```python
from build123d import *

# Parameters (mm, degrees)
SKETCH1_R               = 67
SKETCH1_R_2             = 2.5
BOSS_EXTRUDE1_DEPTH     = 6
CUT_EXTRUDE3_DEPTH      = 47
CUT_EXTRUDE3_DEPTH_BACK = 25
CUT_EXTRUDE6_DEPTH      = 10
CUT_EXTRUDE7_DEPTH      = 10


with BuildPart() as part:
    # Sketch1 → Boss-Extrude1 (new body)
    with BuildSketch(Plane.XY):
        Circle(SKETCH1_R)
        with Locations((0, 58)):
            Circle(SKETCH1_R_2, mode=Mode.SUBTRACT)
        with Locations((58, 0)):
            Circle(SKETCH1_R_2, mode=Mode.SUBTRACT)
        with Locations((0, -58)):
            Circle(SKETCH1_R_2, mode=Mode.SUBTRACT)
        with Locations((-58, 0)):
            Circle(SKETCH1_R_2, mode=Mode.SUBTRACT)
    extrude(amount=BOSS_EXTRUDE1_DEPTH)

    # Sketch3 → Cut-Extrude3 (cut, two sides: drawn at the far end of the back side and taken through both)
    with BuildSketch(Plane.XY.offset(6).offset(-CUT_EXTRUDE3_DEPTH_BACK)):
        Polygon((-34.424621456, -26.646446356), (-27.353553137, -19.575379051), (-19.575378544, -27.353553644), (-26.646446863, -34.424620949), align=None)
        Polygon((19.575379051, 27.353553137), (27.353553644, 19.575378544), (34.424620949, 26.646446863), (26.646446356, 34.424621456), align=None)
    extrude(amount=CUT_EXTRUDE3_DEPTH + CUT_EXTRUDE3_DEPTH_BACK, mode=Mode.SUBTRACT)

    # Sketch4 → Cut-Extrude6 (cut)
    with BuildSketch(Plane.XY.offset(6)):
        Polygon((-19.445436483, 33.587572106), (33.587572106, -19.445436483), (19.445436483, -33.587572106), (-33.587572106, 19.445436483), align=None)
    extrude(amount=-CUT_EXTRUDE6_DEPTH, mode=Mode.SUBTRACT)

    # Sketch5 → Cut-Extrude7 (cut)
    with BuildSketch(Plane.XY.offset(6)):
        Polygon((-34.424621456, -26.646446356), (-34.778174339, -26.292893473), (-27.707106527, -19.221825661), (-27.353553137, -19.575379051), align=None)
        Polygon((-26.646446863, -34.424620949), (-26.292893473, -34.778174339), (-19.221825661, -27.707106527), (-19.575378544, -27.353553644), align=None)
        Polygon((27.707106527, 19.221825661), (27.353553644, 19.575378544), (34.424620949, 26.646446863), (34.778174339, 26.292893473), align=None)
        Polygon((26.646446356, 34.424621456), (19.575379051, 27.353553137), (19.221825661, 27.707106527), (26.292893473, 34.778174339), align=None)
    extrude(amount=-CUT_EXTRUDE7_DEPTH, mode=Mode.SUBTRACT)


solid = part.part
```
The listing builds one solid part. Answer for the finished solid, in the listing's coordinates (mm). A direction names the side the tool comes from. Coordinates: 2 decimals unless noted, no trailing zeros. Loops run counter-clockwise (first coordinate to the right, second up) from the corner with the lowest first, then second, coordinate; pieces in that order, holes last. Notation, with made-up numbers: M 7,-20 L 20,-20 A26 cw 20,5 Z; hole C -23,-40 d8. An arc over 180 degrees is marked long. Answer as CSV lines item,"result". Start each with the question number.
(1) Given pin 1 (2 mm diameter, centred on y = 44, z = 3.5, fed in from +X); pin 2 (1.5 mm diameter, centred on y = -51, z = 5, fed in from +X); pin 3 (1 mm diameter, centred on y = -29, z = 5, fed in from +X), each flat-ended and moving along its own axis, determine where each tip first touches the part or whether it passes through.
(2) The mould has two halves that part along X. Classify faces 3 (the flat face through (6.7, 7.44, 3.04)), 4 (the flat face through (-1, -14, 6)), 5 (the cylindrical face through (-14.524, -65.407, 2.958)): pulls with the +X half, pulls with the -X half, needs draft (parallel to the pull), parting line crosses it, or undercut.
(3) The part is cut by section C-C (y = 58). Give the vertices of the cut face in (x, z).
(4) Find the intervals of material crossed by L1, parallel to Y at x = -29.5, z = 2.5; L2, parallel to X at y = 28.5, z = 4.25; L3, parallel to Y at x = 21, z = 3.75, in increasing order. Write a range as [from, to].
(5) The part is cut by section B-B (x = 0). Give the vertices of the cut face in (y, z).
(6) The part is cut by section A-A (z = 1.5). Give the vertices of the cut face in (x, y).
(7) For faces 1 (the flat face through (-1, -14, 0)), 2 (the flat face through (-31.292, -22.807, 3.042)), determine the directions among +Z, -Z, +X, -X, +Y, -Y from which every point of the face is accessible in a straight line to the end or side of a thin tool.
Determined:
1,pin 1,"x = 51.38"
1,pin 2,"x = 44.32"
1,pin 3,"x = 60.64"
2,face 3,"undercut"
2,face 4,"needs draft"
2,face 5,"parting line crosses it"
3,outline,"M -33.54,0 L -2.5,0 L -2.5,6 L -33.54,6 Z; M 2.5,0 L 33.54,0 L 33.54,6 L 2.5,6 Z"
4,L1,"[-60.16, -31.57], [-21.01, 15.36], [23.53, 60.16]"
4,L2,"[-60.64, -24.53], [-14.36, 20.01], [32.57, 60.64]"
4,L3,"[-63.62, -32.03], [-6.86, 25.93], [29.49, 63.62]"
5,outline,"M -67,0 L -60.5,0 L -60.5,6 L -67,6 Z; M -55.5,0 L -14.14,0 L -14.14,6 L -55.5,6 Z; M 14.14,0 L 55.5,0 L 55.5,6 L 14.14,6 Z; M 60.5,0 L 67,0 L 67,6 L 60.5,6 Z"
6,outline,"C 0,0 d134; hole C -58,0 d5; hole M -34.78,-26.29 L -26.29,-34.78 L -19.22,-27.71 L -27.71,-19.22 Z; hole M -33.59,19.45 L 19.45,-33.59 L 33.59,-19.45 L -19.45,33.59 Z; hole C 0,-58 d5; hole C 0,58 d5; hole M 19.22,27.71 L 27.71,19.22 L 34.78,26.29 L 26.29,34.78 Z; hole C 58,0 d5"
7,face 1,"-Z, +X, -X, +Y, -Y"
7,face 2,"+Z, -Z"
